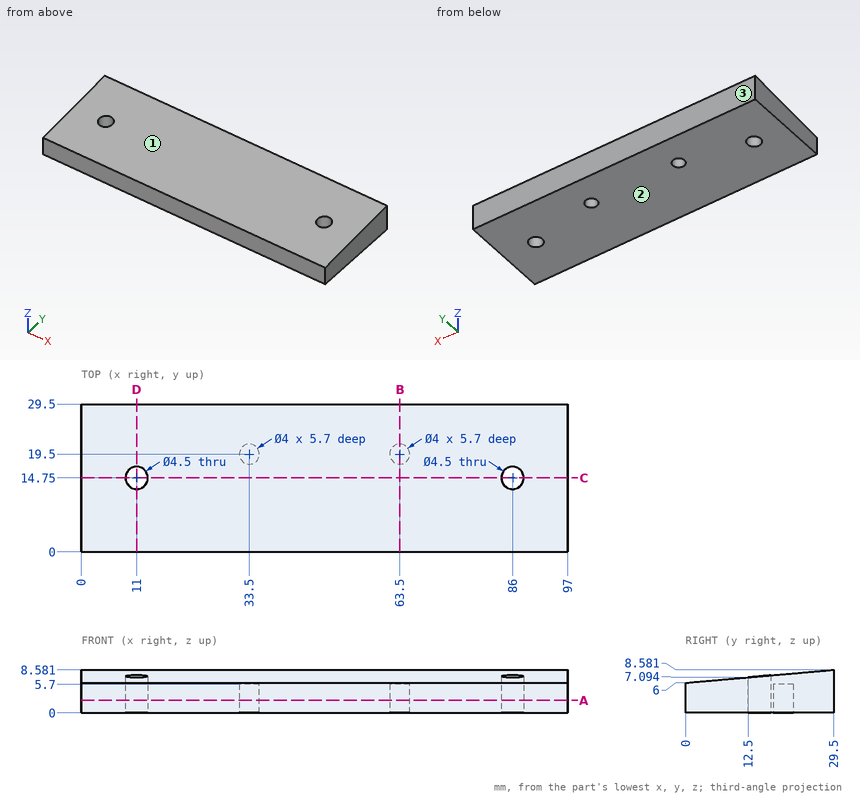
Study the drawing (mm; zero at the part's minimum x, y, z) and answer. Give positions to 0.01 mm unless a question says otherwise; leave off trailing zeros. Write each loop counter-clockwise with the first axis right and the second up, starting at its lowest first coordinate (ties: lowest second). Pieces come first, ordered by that corner, then holes.
(1) The part is cut by section C-C on y = 14.75. Write down the section's boundary in (x, z).
Final values:
outline: (0, 0) - (8.75, 0) - (8.75, 7.29) - (0, 7.29) - close; (13.25, 0) - (83.75, 0) - (83.75, 7.29) - (13.25, 7.29) - close; (88.25, 0) - (97, 0) - (97, 7.29) - (88.25, 7.29) - close
(2) The part is cut by section D-D on x = 11. Write down the section's boundary in (y, z), plus the area to 3 significant figures.
Final values:
outline: (0, 0) - (12.5, 0) - (12.5, 7.09) - (0, 6) - close; (17, 0) - (29.5, 0) - (29.5, 8.58) - (17, 7.49) - close
area: 182 mm2
(3) Flat-ended cylindrical pins translate along their axes: pin 1 Ø1.2 at (x, y) = (64, 20.5) entering from -Z; pin 2 Ø2.5 at (x, y) = (86, 14.75) entering from -Z; pin 3 Ø12 at (x, y) = (60, 13) entering from +Z; pin 4 Ø3.5 at (x, y) = (63.5, 19.5) entering from +Z. Find the tip coordinate at first contact, or state that the pin passes through.
Final values:
pin 1: stops at z = 5.7
pin 2: passes through
pin 3: stops at z = 7.66
pin 4: stops at z = 7.86
(4) The mould has two halves that part along Z. Classify the marked faces 1, 2 and 3: pulls with the +Z half, pulls with the -Z half, needs draft (parallel to the pull), parting line crosses it, or undercut.
Final values:
face 1: pulls with the +Z half
face 2: pulls with the -Z half
face 3: needs draft
(5) The part is cut by section A-A on z = 2.5. Write down the section's boundary in (x, y), plus the area to 3 significant figures.
Final values:
outline: (0, 0) - (97, 0) - (97, 29.5) - (0, 29.5) - close; hole circle Ø4.5 at (11, 14.75); hole circle Ø4 at (33.5, 19.5); hole circle Ø4 at (63.5, 19.5); hole circle Ø4.5 at (86, 14.75)
area: 2,800 mm2
(6) Straight lines are drawn through the part: line 1 (X direction, y = 14.75, z = 4.25); line 2 (Y direction, x = 63.5, z = 3.45); line 3 (Y direction, x = 84, z = 4.75). For each, find the intervals that lie inside material, in ascending order.
Final values:
line 1: x = 0 to 8.75, 13.25 to 83.75, 88.25 to 97
line 2: y = 0 to 17.5, 21.5 to 29.5
line 3: y = 0 to 13.72, 15.78 to 29.5
(7) The part is cut by section B-B on x = 63.5. Write down the section's boundary in (y, z), plus the area to 3 significant figures.
Final values:
outline: (0, 0) - (17.5, 0) - (17.5, 5.7) - (21.5, 5.7) - (21.5, 0) - (29.5, 0) - (29.5, 8.58) - (0, 6) - close
area: 192 mm2
